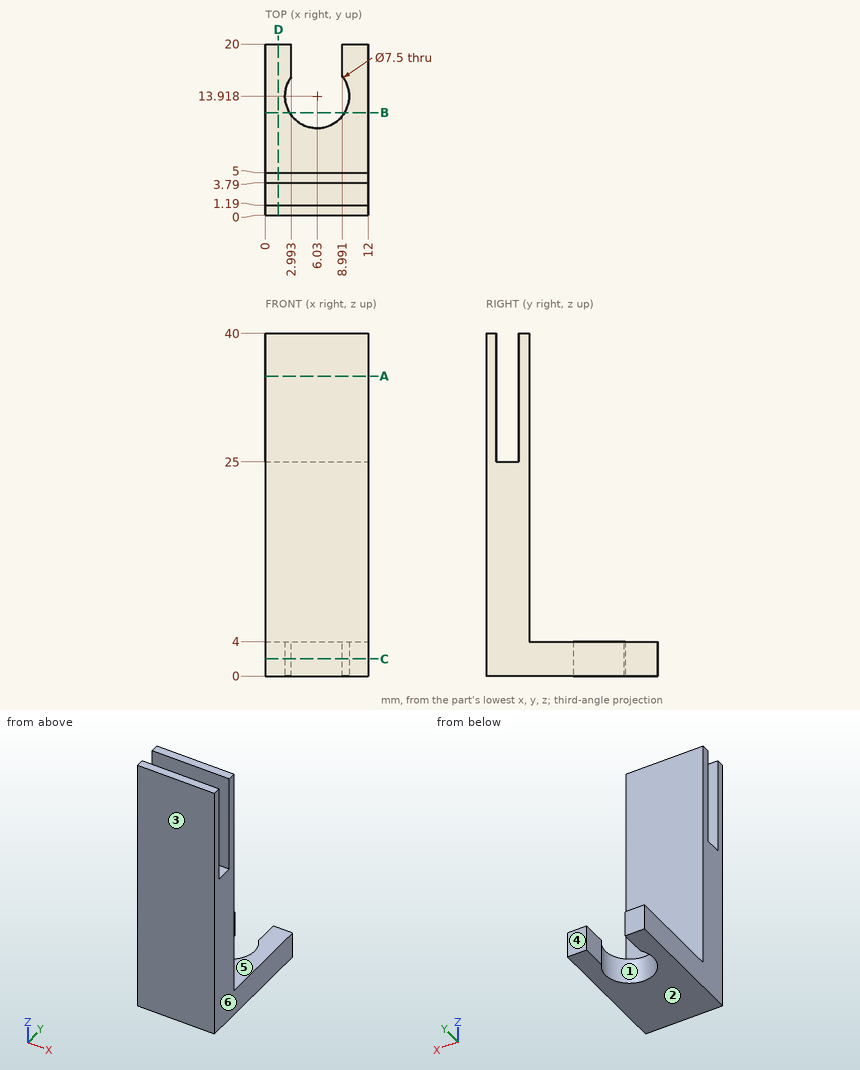
Could you check a few things on this drawing? It's one solid part, dimensions in mm from its lowest x, y, z. A direction names the side the tool comes from. Coordinates: 2 decimals unless noted, no trailing zeros. Write each loop counter-clockwise with the first axis right and the second up, starting at its lowest first coordinate (ties: lowest second). Pieces come first, ordered by that corner, then holes.
Q1. Please list where these lines run through material, in increasing order: L1, parallel to Y at x = 3.25, z = 29; L2, parallel to Y at x = 8, z = 10.5; L3, parallel to Z at x = 4.5, y = 7.5.
Results found:
L1: y = 0 to 1.19, 3.79 to 5
L2: y = 0 to 5
L3: z = 0 to 4
Q2. For P1, Ø0.8, axis at x = 6, y = 2.5, coming from the +Z side; P2, Ø6, axis at x = 10, z = 13.5, coming from the +Y side, each with a flat end and sliding along its axis, tell me the tip position at first contact or that it passes through.
Results found:
P1: stops at z = 25
P2: stops at y = 5
Q3. If we mould it in two halves opening along Y, with no side actions, what happens to the marked faces 1, 2, 3 and 4? For each: +Y half, -Y half, draft (parallel to the pull), parting line (faces both ways), or undercut.
Results found:
face 1: undercut
face 2: draft
face 3: -Y half
face 4: +Y half
Q4. Imagine slicing it at B-B, the plane y = 12. List the corners of the cut face in (x, z) for me.
Results found:
outline: (0, 0) - (2.81, 0) - (2.81, 4) - (0, 4) - close; (9.25, 0) - (12, 0) - (12, 4) - (9.25, 4) - close
Q5. Imagine slicing it at D-D, the plane x = 1.5. List the corners of the cut face in (y, z) for me, plus the area to 3 significant figures.
Results found:
outline: (0, 0) - (20, 0) - (20, 4) - (5, 4) - (5, 40) - (3.79, 40) - (3.79, 25) - (1.19, 25) - (1.19, 40) - (0, 40) - close
area: 221 mm2
Q6. Imagine slicing it at C-C, the plane z = 2. List the corners of the cut face in (x, y) for me, plus the area to 3 significant figures.
Results found:
outline: (0, 0) - (12, 0) - (12, 20) - (8.99, 20) - (8.99, 16.22) arc R3.75 cw (long way) to (2.99, 16.12) - (2.99, 20) - (0, 20) - close
area: 179 mm2
Q7. Which directions (+Z, -Z, +X, -X, +Y, -Y) give clear straight access to the entire face, cutting with the end or side of a thin tool? Please do the marked faces 5 and 6.
Results found:
face 5: +Z, +X, -X, +Y
face 6: +Z, -Z, +X, +Y, -Y
Q8. Imagine slicing it at A-A, the plane z = 35. List the corners of the cut face in (x, y) for me.
Results found:
outline: (0, 0) - (12, 0) - (12, 1.19) - (0, 1.19) - close; (0, 3.79) - (12, 3.79) - (12, 5) - (0, 5) - close
